Part model, mm, in its own coordinate system. Face numbers are marked on the shaded views. A direction names the side the tool comes from. Coordinates: 2 decimals unless noted, no trailing zeros. Write each loop counter-clockwise with the first axis right and the second up, starting at its lowest first coordinate (ties: lowest second). Pieces come first, ordered by that corner, then holes. Notation, with made-up numbers: (17.25, 12.25) -> (47.25, 12.25) arc R22 ccw to (47.25, 31.25) -> close; hole circle Ø6 at (83, 48). An arc over 180 degrees is marked (long way). Write item = value, one per line.
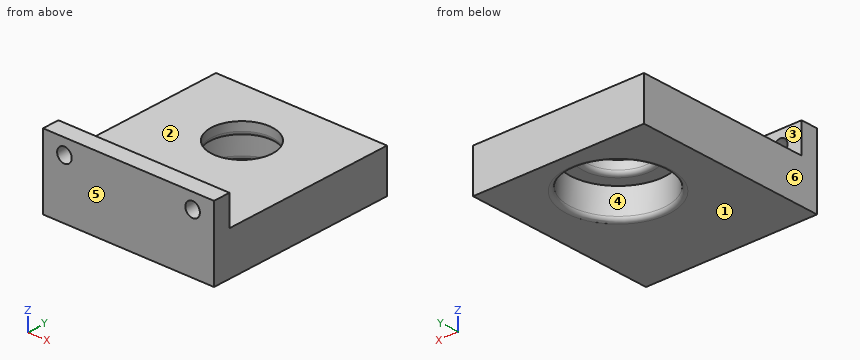
from build123d import *

# Parameters (mm, degrees)
SKETCH1_W           = 40
SKETCH1_H           = 45
SKETCH1_R           = 11.15
BOSS_EXTRUDE1_DEPTH = 7
SKETCH2_W           = 40
SKETCH2_H           = 45
SKETCH2_R           = 7.15
BOSS_EXTRUDE2_DEPTH = 3
FILLET1_R           = 1
SKETCH3_W           = 40
SKETCH3_H           = 4
BOSS_EXTRUDE3_DEPTH = 7
SKETCH4_R           = 1.7
CUT_EXTRUDE1_DEPTH  = 49.682645779


with BuildPart() as part:
    # Sketch1 → Boss-Extrude1 (new body)
    with BuildSketch(Plane.XY):
        Rectangle(SKETCH1_W, SKETCH1_H)
        with Locations((0, 7)):
            Circle(SKETCH1_R, mode=Mode.SUBTRACT)
    extrude(amount=BOSS_EXTRUDE1_DEPTH)

    # Sketch2 → Boss-Extrude2 (add)
    with BuildSketch(Plane.XY.offset(7)):
        Rectangle(SKETCH2_W, SKETCH2_H)
        with Locations((0, 7)):
            Circle(SKETCH2_R, mode=Mode.SUBTRACT)
    extrude(amount=BOSS_EXTRUDE2_DEPTH)

    # Fillet1
    fillet1_edges = [part.edges().sort_by_distance(p)[0] for p in [
        (-11.15, 7, 0),
        (-7.15, 7, 7),
    ]]
    fillet(fillet1_edges, radius=FILLET1_R)

    # Sketch3 → Boss-Extrude3 (add)
    with BuildSketch(Plane.XY.offset(10)):
        with Locations((0, -20.5)):
            Rectangle(SKETCH3_W, SKETCH3_H)
    extrude(amount=BOSS_EXTRUDE3_DEPTH)

    # Sketch4 → Cut-Extrude1 (cut, through all)
    with BuildSketch(Plane(origin=(0, -18.5, 0), x_dir=(1, 0, 0), z_dir=(0, 1, 0))):
        with Locations(Location((-15, -13.5, 0), (0, 0, 270))):
            Circle(SKETCH4_R)
        with Locations(Location((15, -13.5, 0), (0, 0, 270))):
            Circle(SKETCH4_R)
    extrude(amount=-CUT_EXTRUDE1_DEPTH, mode=Mode.SUBTRACT)


solid = part.part
Q1. Saw through at D-D on x = 0. Give the cut face in (y, z).
Model answer:
outline = (-22.5, 0) -> (-5.15, 0) arc R1 ccw to (-4.15, 1) -> (-4.15, 7) -> (-1.15, 7) arc R1 ccw to (-0.15, 8) -> (-0.15, 10) -> (-18.5, 10) -> (-18.5, 17) -> (-22.5, 17) -> close; (14.15, 8) arc R1 ccw to (15.15, 7) -> (18.15, 7) -> (18.15, 1) arc R1 ccw to (19.15, 0) -> (22.5, 0) -> (22.5, 10) -> (14.15, 10) -> close
Q2. Saw through at C-C on z = 5.5. Give the cut face in (x, y).
Model answer:
outline = (-20, -22.5) -> (20, -22.5) -> (20, 22.5) -> (-20, 22.5) -> close; hole circle Ø22.3 at (0, 7)
Q3. Mould opens along Y. For the marked faces 3, 4, 5 and 6 say: released by +Y, released by -Y, zero draft, split by the parting line, or undercut.
Model answer:
face_3 = released by +Y
face_4 = undercut
face_5 = released by -Y
face_6 = zero draft
Q4. Pin check, flat tips, straight feed: pin 1 (18 mm diameter, centred on x = 0, y = 7, fed in from -Z); pin 2 (12 mm diameter, centred on x = -2.5, y = -1, fed in from +Z); pin 3 (2 mm diameter, centred on x = -9.5, z = 12, fed in from +Y). Stop position of each tip, or through.
Model answer:
pin_1 = 7
pin_2 = 10
pin_3 = -18.5
Q5. Which spindle directions (+Z, -Z, +X, -X, +Y, -Y) get a long thin tool onto all of the face, cutting with end or side? Do the marked faces 1 and 2. Say none if no direction does.
Model answer:
face_1 = -Z, +X, -X, +Y, -Y
face_2 = +Z, +X, -X, +Y
Q6. Saw through at A-A on y = 7. Give the cut face in (x, z), and give its area (3 significant figures).
Model answer:
outline = (-20, 0) -> (-12.15, 0) arc R1 ccw to (-11.15, 1) -> (-11.15, 7) -> (-8.15, 7) arc R1 ccw to (-7.15, 8) -> (-7.15, 10) -> (-20, 10) -> close; (7.15, 8) arc R1 ccw to (8.15, 7) -> (11.15, 7) -> (11.15, 1) arc R1 ccw to (12.15, 0) -> (20, 0) -> (20, 10) -> (7.15, 10) -> close
area = 200 mm²
Q7. Probe line 1 (X direction, y = -21.5, z = 13.5); line 2 (Y direction, x = 0, z = 6.75); line 3 (Y direction, x = 0, z = 8.95). List the from-to ranges inside material, lowest first. Write a range as from..to.
Model answer:
line_1 = -20..-16.7, -13.3..13.3, 16.7..20
line_2 = -22.5..-4.15, 18.15..22.5
line_3 = -22.5..-0.15, 14.15..22.5
Q8. Saw through at B-B on x = 15. Give the cut face in (y, z).
Model answer:
outline = (-22.5, 0) -> (22.5, 0) -> (22.5, 10) -> (-18.5, 10) -> (-18.5, 11.8) -> (-22.5, 11.8) -> close; (-22.5, 15.2) -> (-18.5, 15.2) -> (-18.5, 17) -> (-22.5, 17) -> close
